Here's how the part is built. I have some questions about the finished solid (model axes, mm). A direction names the side the tool comes from. Give positions to 0.01 mm unless a question says otherwise; leave off trailing zeros. Loops run counter-clockwise (first coordinate to the right, second up) from the corner with the lowest first, then second, coordinate; pieces in that order, holes last.
Q1. We'd pull the mould along X, two halves only. Please class faces 4 (the face through (-37, 17, 0)), 5 (the face through (0, 18, 22.5)), 6 (the face through (36, 17, -14)), 7 (the face through (37, 17, 0)): +X half, -X half, draft (parallel to the pull), parting line (faces both ways), or undercut.
Q2. If we section it at C-C (y = 16): Please give me the cut outline in (x, z).
Q3. I need wall thicknesses on line 1 (Z direction, x = -12, y = 20); line 2 (X direction, y = 14, z = 6.5); line 3 (X direction, y = 32.5, z = -4.5). Which ranges of each line are inside material? Lowest first, please.
Q4. For faces 1 (the face through (-1, 17, 24)), 2 (the face through (36, 12, -11)), 3 (the face through (0, 18, -22.5)), which set-ups out of +Z, -Z, +X, -X, +Y, -Y let a thin tool reach every point of the face, with its end or its side?
Q5. Will this pin go through, and if not, where does the flat tip stop? P1, Ø23, axis at x = 6, z = 10, coming from the +Y side.
Q6. If we section it at B-B (z = 11): Please give me the cut outline in (x, y), plus the area to 3 significant figures.
Q7. If we section it at A-A (y = 26.5): Please give me the cut outline in (x, z).
from build123d import *

# Parameters (mm, degrees)
SKETCH1_W           = 74
SKETCH1_H           = 48
BOSS_EXTRUDE1_DEPTH = 34
SKETCH3_W           = 71
SKETCH3_H           = 45
CUT_EXTRUDE1_DEPTH  = 31
SKETCH4_W           = 72.185535561
SKETCH4_H           = 46.080093343
CUT_EXTRUDE2_DEPTH  = 2
SKETCH5_W           = 6
SKETCH5_H           = 10
CUT_EXTRUDE3_DEPTH  = 5


with BuildPart() as part:
    # Sketch1 → Boss-Extrude1 (new body)
    with BuildSketch(Plane(origin=(0, 0, 0), x_dir=(1, 0, 0), z_dir=(0, 1, 0))):
        Rectangle(SKETCH1_W, SKETCH1_H)
    extrude(amount=BOSS_EXTRUDE1_DEPTH)

    # Sketch3 → Cut-Extrude1 (cut)
    with BuildSketch(Plane(origin=(0, 34, 0), x_dir=(1, 0, 0), z_dir=(0, 1, 0))):
        Rectangle(SKETCH3_W, SKETCH3_H)
    extrude(amount=-CUT_EXTRUDE1_DEPTH, mode=Mode.SUBTRACT)

    # Sketch4 → Cut-Extrude2 (cut)
    with BuildSketch(Plane(origin=(0, 34, 0), x_dir=(1, 0, 0), z_dir=(0, 1, 0))):
        with Locations((0.092767781, 0.040046672)):
            Rectangle(SKETCH4_W, SKETCH4_H)
    extrude(amount=-CUT_EXTRUDE2_DEPTH, mode=Mode.SUBTRACT)

    # Sketch5 → Cut-Extrude3 (cut)
    with BuildSketch(Plane(origin=(37, 0, 0), x_dir=(0, 0, -1), z_dir=(1, 0, 0))):
        with Locations((11, 17)):
            Rectangle(SKETCH5_W, SKETCH5_H)
    extrude(amount=-CUT_EXTRUDE3_DEPTH, mode=Mode.SUBTRACT)


solid = part.part
Check sheet entries:
1. face 4: -X half
1. face 5: undercut
1. face 6: draft
1. face 7: +X half
2. outline: (-37, -24) - (37, -24) - (37, -14) - (35.5, -14) - (35.5, -22.5) - (-35.5, -22.5) - (-35.5, 22.5) - (35.5, 22.5) - (35.5, -8) - (37, -8) - (37, 24) - (-37, 24) - close
3. line 1: z = -24 to -22.5, 22.5 to 24
3. line 2: x = -37 to -35.5, 35.5 to 37
3. line 3: x = -37 to -36, 36.19 to 37
4. face 1: +Z, +X, -X, +Y, -Y
4. face 2: +X
4. face 3: +Y
5. P1: stops at y = 3
6. outline: (-37, 0) - (37, 0) - (37, 34) - (36.19, 34) - (36.19, 32) - (35.5, 32) - (35.5, 3) - (-35.5, 3) - (-35.5, 32) - (-36, 32) - (-36, 34) - (-37, 34) - close
6. area: 313 mm2
7. outline: (-37, -24) - (37, -24) - (37, 24) - (-37, 24) - close; hole (-35.5, -22.5) - (35.5, -22.5) - (35.5, 22.5) - (-35.5, 22.5) - close
